The listing builds one solid part. Answer for the finished solid, in the listing's coordinates (mm). A direction names the side the tool comes from. Coordinates: 2 decimals unless noted, no trailing zeros. Loops run counter-clockwise (first coordinate to the right, second up) from the corner with the lowest first, then second, coordinate; pieces in that order, holes last. Notation, with made-up numbers: M 79.25,2 L 88.25,2 A11 ccw 88.25,8 Z; hole C 48,76 d5. An arc over 180 degrees is marked long. Return JSON: item names as keys, results as strings. Group by question number.
1. Straight lines are drawn through the part: L1, parallel to X at y = 24.9, z = 0; L2, parallel to X at y = 22.3, z = 23.57; L3, parallel to Y at x = -10.5, z = 25.5. For each, find the intervals that lie inside material, in ascending order. Write a range as from..to.
2. Given P1, Ø3, axis at x = 7.5, y = -17, coming from the +Z side; P2, Ø6, axis at x = -23.57, z = -23.57, coming from the +Y side; P3, Ø4, axis at y = 24.5, z = -6.5, coming from the +X side, each flat-ended and moving along its own axis, determine where each tip first touches the part or whether it passes through.
3. Section D-D (x = 22.5) is taken. Count the separate pieces of the cut face and the enclosed holes in it, then the cut area to 3 significant figures.
4. Section A-A (y = -8) is taken. Write down the section's boundary in (x, z), then the cut area to 3 significant figures.
5. Which of the six approach directions +Z, -Z, +X, -X, +Y, -Y give full straight-line access (tool end or side, diameter ignored) to faces 1 (the face through (20.624, 3.121, 20.532)), 2 (the face through (1.802, 25.289, 5.723)), 3 (the face through (0, -13, -31))?
6. The mould has two halves that part along X. Classify faces 4 (the face through (25.79, 22.13, 22.42)), 5 (the face through (-20.624, 3.121, -20.532)), 6 (the face through (-0.4, 24.5, -19.2)): pulls with the +X half, pulls with the -X half, needs draft (parallel to the pull), parting line crosses it, or undercut.
7. Section C-C (x = 12.5) is taken. Write down the section's boundary in (y, z), then the cut area to 3 significant figures.
```python
from build123d import *

# Parameters (mm, degrees)
SKETCH1_W                = 56.4
SKETCH1_H                = 56.4
BOSS_EXTRUDE1_DEPTH      = 24.5
CUT_EXTRUDE1_START       = 4.8
CUT_EXTRUDE1_DEPTH       = 59.378160784
FILLET1_R                = 3
FILLET2_R                = 1
SKETCH3_R                = 2.5
CUT_EXTRUDE2_DEPTH       = 55.8
SKETCH4_R                = 19.05
BOSS_EXTRUDE2_DEPTH      = 1.6
SKETCH5_R                = 3.175
BOSS_EXTRUDE3_DEPTH      = 33.5
CUT_EXTRUDE3_START       = -15
CUT_EXTRUDE3_DEPTH       = 15
CUT_EXTRUDE4_DEPTH       = 71.388067171
CUT_EXTRUDE4_DEPTH_BACK  = 71.388067171
FILLET3_R                = 5
CUT_EXTRUDE5_START       = -1.6
SKETCH8_R                = 6
SKETCH8_R_2              = 3.175
CUT_EXTRUDE5_DEPTH       = 1.6
BOSS_EXTRUDE4_START      = -11.5
BOSS_EXTRUDE4_DEPTH      = 33
BOSS_EXTRUDE5_DEPTH      = 6.4
BOSS_EXTRUDE5_DEPTH_BACK = 50.6
SKETCH11_R               = 4
BOSS_EXTRUDE6_START      = -1
SKETCH12_W               = 20.6
SKETCH12_H               = 11.5
BOSS_EXTRUDE6_DEPTH      = 6.4


with BuildPart() as part:
    # Sketch1 → Boss-Extrude1 (new, symmetric)
    with BuildSketch(Plane(origin=(0, 0, 0), x_dir=(1, 0, 0), z_dir=(0, 1, 0))):
        Rectangle(SKETCH1_W, SKETCH1_H)
    extrude(amount=BOSS_EXTRUDE1_DEPTH, both=True)

    # Sketch2 → Cut-Extrude1 (cut, through all)
    with BuildSketch(Plane.XZ.offset(-24.5).offset(CUT_EXTRUDE1_START)):
        with BuildLine():
            Line((-18.75, 28.2), (-18.75, 24.75))
            ThreePointArc((-18.75, 24.75), (-20.507359313, 20.507359313), (-24.75, 18.75))
            Line((-24.75, 18.75), (-28.2, 18.75))
            Line((-28.2, 18.75), (-28.2, 28.2))
            Line((-28.2, 28.2), (-18.75, 28.2))
        make_face()
        with BuildLine():
            Line((28.2, 28.2), (28.2, 18.75))
            Line((28.2, 18.75), (24.75, 18.75))
            ThreePointArc((24.75, 18.75), (20.507359313, 20.507359313), (18.75, 24.75))
            Line((18.75, 24.75), (18.75, 28.2))
            Line((18.75, 28.2), (28.2, 28.2))
        make_face()
        with BuildLine():
            Line((18.75, -28.2), (18.75, -24.75))
            ThreePointArc((18.75, -24.75), (20.507359313, -20.507359313), (24.75, -18.75))
            Line((24.75, -18.75), (28.2, -18.75))
            Line((28.2, -18.75), (28.2, -28.2))
            Line((28.2, -28.2), (18.75, -28.2))
        make_face()
        with BuildLine():
            Line((-28.2, -28.2), (-28.2, -18.75))
            Line((-28.2, -18.75), (-24.75, -18.75))
            ThreePointArc((-24.75, -18.75), (-20.507359313, -20.507359313), (-18.75, -24.75))
            Line((-18.75, -24.75), (-18.75, -28.2))
            Line((-18.75, -28.2), (-28.2, -28.2))
        make_face()
    extrude(amount=CUT_EXTRUDE1_DEPTH, mode=Mode.SUBTRACT)

    # Fillet1
    fillet1_edges = [part.edges().sort_by_distance(p)[0] for p in [
        (-28.2, -2.4, -18.75),
        (-18.75, -2.4, -28.2),
        (18.75, -2.4, -28.2),
        (28.2, -2.4, -18.75),
        (28.2, -2.4, 18.75),
        (18.75, -2.4, 28.2),
        (-18.75, -2.4, 28.2),
        (-28.2, -2.4, 18.75),
        (28.2, 22.1, 28.2),
        (-28.2, 22.1, 28.2),
        (-28.2, 22.1, -28.2),
        (28.2, 22.1, -28.2),
    ]]
    fillet(fillet1_edges, radius=FILLET1_R)

    # Fillet2
    fillet2_edges = [part.edges().sort_by_distance(p)[0] for p in [
        (-20.507359313, -24.5, -20.507359313),
        (-24.975, -24.5, -18.75),
        (20.507359313, -24.5, -20.507359313),
        (18.75, -24.5, -24.975),
        (20.507359313, -24.5, 20.507359313),
        (24.975, -24.5, 18.75),
        (-20.507359313, -24.5, 20.507359313),
        (-18.75, -24.5, 24.975),
        (-28.2, -24.5, 0),
        (-18.75, -24.5, -24.975),
        (0, -24.5, -28.2),
        (24.975, -24.5, -18.75),
        (28.2, -24.5, 0),
        (18.75, -24.5, 24.975),
        (0, -24.5, 28.2),
        (-24.975, -24.5, 18.75),
        (-17.871320344, -24.5, 27.321320344),
        (-17.871320344, -24.5, -27.321320344),
        (17.871320344, -24.5, -27.321320344),
        (27.321320344, -24.5, -17.871320344),
        (27.321320344, -24.5, 17.871320344),
        (17.871320344, -24.5, 27.321320344),
        (-27.321320344, -24.5, 17.871320344),
        (-27.321320344, -24.5, -17.871320344),
    ]]
    fillet(fillet2_edges, radius=FILLET2_R)

    # Sketch3 → Cut-Extrude2 (cut)
    with BuildSketch(Plane(origin=(0, 24.5, 0), x_dir=(1, 0, 0), z_dir=(0, 1, 0))):
        with Locations(Location((23.57, 23.57, 0), (0, 0, 270))):
            Circle(SKETCH3_R)
        with Locations(Location((-23.57, 23.57, 0), (0, 0, 90))):
            Circle(SKETCH3_R)
        with Locations(Location((23.57, -23.57, 0), (0, 0, 90))):
            Circle(SKETCH3_R)
        with Locations(Location((-23.57, -23.57, 0), (0, 0, 270))):
            Circle(SKETCH3_R)
    extrude(amount=-CUT_EXTRUDE2_DEPTH, mode=Mode.SUBTRACT)

    # Sketch4 → Boss-Extrude2 (add)
    with BuildSketch(Plane(origin=(0, 24.5, 0), x_dir=(1, 0, 0), z_dir=(0, 1, 0))):
        with Locations(Location((0, 0, 0), (0, 0, 270))):
            Circle(SKETCH4_R)
    extrude(amount=BOSS_EXTRUDE2_DEPTH)

    # Sketch5 → Boss-Extrude3 (add)
    with BuildSketch(Plane(origin=(0, 24.5, 0), x_dir=(1, 0, 0), z_dir=(0, 1, 0))):
        with Locations(Location((0, 0, 0), (0, 0, 270))):
            Circle(SKETCH5_R)
    extrude(amount=BOSS_EXTRUDE3_DEPTH)

    # Sketch6 → Cut-Extrude3 (cut)
    with BuildSketch(Plane(origin=(0, 58, 0), x_dir=(1, 0, 0), z_dir=(0, 1, 0)).offset(CUT_EXTRUDE3_START)):
        with BuildLine():
            Line((-2.049390153, 2.425), (2.049390153, 2.425))
            ThreePointArc((2.049390153, 2.425), (0, 3.175), (-2.049390153, 2.425))
        make_face()
    extrude(amount=CUT_EXTRUDE3_DEPTH, mode=Mode.SUBTRACT)

    # Sketch7 → Cut-Extrude4 (cut, two sides: drawn at the far end of the back side and taken through both)
    with BuildSketch(Plane(origin=(0, 0, 0), x_dir=(0, 0, -1), z_dir=(1, 0, 0)).offset(-CUT_EXTRUDE4_DEPTH_BACK)):
        Polygon((2.425, 43), (3.175, 41), (3.175, 43), align=None)
    extrude(amount=CUT_EXTRUDE4_DEPTH + CUT_EXTRUDE4_DEPTH_BACK, mode=Mode.SUBTRACT)

    # Fillet3
    fillet3_edges = [part.edges().sort_by_distance(p)[0] for p in [
        (0, 43, -2.425),
    ]]
    fillet(fillet3_edges, radius=FILLET3_R)

    # Sketch8 → Cut-Extrude5 (cut)
    with BuildSketch(Plane(origin=(0, 26.1, 0), x_dir=(1, 0, 0), z_dir=(0, 1, 0)).offset(CUT_EXTRUDE5_START)):
        with Locations(Location((0, 0, 0), (0, 0, 270))):
            Circle(SKETCH8_R)
        with Locations(Location((0, 0, 0), (0, 0, 59.774237817))):
            Circle(SKETCH8_R_2, mode=Mode.SUBTRACT)
    extrude(amount=CUT_EXTRUDE5_DEPTH, mode=Mode.SUBTRACT)

    # Sketch11 → Boss-Extrude5 (add, two sides: drawn at the far end of the back side and taken through both)
    with BuildSketch(Plane(origin=(0, 26.1, 0), x_dir=(1, 0, 0), z_dir=(0, 1, 0)).offset(-BOSS_EXTRUDE5_DEPTH_BACK)):
        with Locations(Location((0, 0, 0), (0, 0, 270))):
            Circle(SKETCH11_R)
    extrude(amount=BOSS_EXTRUDE5_DEPTH + BOSS_EXTRUDE5_DEPTH_BACK)



with BuildPart() as body_2:
    # Sketch10 → Boss-Extrude4 (new body)
    with BuildSketch(Plane.XZ.offset(24.5).offset(BOSS_EXTRUDE4_START)):
        with BuildLine():
            Line((25.2, 18.85), (24.75, 18.85))
            ThreePointArc((24.75, 18.85), (20.578069991, 20.578069991), (18.85, 24.75))
            Line((18.85, 24.75), (18.85, 25.2))
            ThreePointArc((18.85, 25.2), (17.942031022, 27.392031022), (15.75, 28.3))
            Line((15.75, 28.3), (-15.75, 28.3))
            ThreePointArc((-15.75, 28.3), (-17.942031022, 27.392031022), (-18.85, 25.2))
            Line((-18.85, 25.2), (-18.85, 24.75))
            ThreePointArc((-18.85, 24.75), (-20.578069991, 20.578069991), (-24.75, 18.85))
            Line((-24.75, 18.85), (-25.2, 18.85))
            ThreePointArc((-25.2, 18.85), (-27.392031022, 17.942031022), (-28.3, 15.75))
            Line((-28.3, 15.75), (-28.3, -15.75))
            ThreePointArc((-28.3, -15.75), (-27.392031022, -17.942031022), (-25.2, -18.85))
            Line((-25.2, -18.85), (-24.75, -18.85))
            ThreePointArc((-24.75, -18.85), (-20.578069991, -20.578069991), (-18.85, -24.75))
            Line((-18.85, -24.75), (-18.85, -25.2))
            ThreePointArc((-18.85, -25.2), (-17.942031022, -27.392031022), (-15.75, -28.3))
            Line((-15.75, -28.3), (15.75, -28.3))
            ThreePointArc((15.75, -28.3), (17.942031022, -27.392031022), (18.85, -25.2))
            Line((18.85, -25.2), (18.85, -24.75))
            ThreePointArc((18.85, -24.75), (20.578069991, -20.578069991), (24.75, -18.85))
            Line((24.75, -18.85), (25.2, -18.85))
            ThreePointArc((25.2, -18.85), (27.392031022, -17.942031022), (28.3, -15.75))
            Line((28.3, -15.75), (28.3, 15.75))
            ThreePointArc((28.3, 15.75), (27.392031022, 17.942031022), (25.2, 18.85))
        make_face()
        with BuildLine():
            Line((28.2, -15.75), (28.2, 15.75))
            ThreePointArc((28.2, 15.75), (27.321320344, 17.871320344), (25.2, 18.75))
            Line((25.2, 18.75), (24.75, 18.75))
            ThreePointArc((24.75, 18.75), (20.507359313, 20.507359313), (18.75, 24.75))
            Line((18.75, 24.75), (18.75, 25.2))
            ThreePointArc((18.75, 25.2), (17.871320344, 27.321320344), (15.75, 28.2))
            Line((15.75, 28.2), (-15.75, 28.2))
            ThreePointArc((-15.75, 28.2), (-17.871320344, 27.321320344), (-18.75, 25.2))
            Line((-18.75, 25.2), (-18.75, 24.75))
            ThreePointArc((-18.75, 24.75), (-20.507359313, 20.507359313), (-24.75, 18.75))
            Line((-24.75, 18.75), (-25.2, 18.75))
            ThreePointArc((-25.2, 18.75), (-27.321320344, 17.871320344), (-28.2, 15.75))
            Line((-28.2, 15.75), (-28.2, -15.75))
            ThreePointArc((-28.2, -15.75), (-27.321320344, -17.871320344), (-25.2, -18.75))
            Line((-25.2, -18.75), (-24.75, -18.75))
            ThreePointArc((-24.75, -18.75), (-20.507359313, -20.507359313), (-18.75, -24.75))
            Line((-18.75, -24.75), (-18.75, -25.2))
            ThreePointArc((-18.75, -25.2), (-17.871320344, -27.321320344), (-15.75, -28.2))
            Line((-15.75, -28.2), (15.75, -28.2))
            ThreePointArc((15.75, -28.2), (17.871320344, -27.321320344), (18.75, -25.2))
            Line((18.75, -25.2), (18.75, -24.75))
            ThreePointArc((18.75, -24.75), (20.507359313, -20.507359313), (24.75, -18.75))
            Line((24.75, -18.75), (25.2, -18.75))
            ThreePointArc((25.2, -18.75), (27.321320344, -17.871320344), (28.2, -15.75))
        make_face(mode=Mode.SUBTRACT)
    extrude(amount=-BOSS_EXTRUDE4_DEPTH)


with BuildPart() as part_1:
    add(part.part)

    add(body_2.part)  # Boss-Extrude6 merges body 2
    # Sketch12 → Boss-Extrude6 (add)
    with BuildSketch(Plane(origin=(0, 0, -28.2), x_dir=(-1, 0, 0), z_dir=(0, 0, -1)).offset(BOSS_EXTRUDE6_START)):
        with Locations((0, -18.75)):
            Rectangle(SKETCH12_W, SKETCH12_H)
    extrude(amount=BOSS_EXTRUDE6_DEPTH)


solid = part_1.part
```
Worked out:
{
 "1": {"L1": "-19.05..-6, -4..4, 6..19.05", "L2": "-28.2..-26.07, -21.07..21.07, 26.07..28.2", "L3": "-24.5..24.5"},
 "2": {"P1": "z = 28.2", "P2": "y = 24.5", "P3": "x = 28.2"},
 "3": {"separate pieces": "3", "enclosed holes": "0", "area": "1,930 mm^2"},
 "4": {"outline": "M -28.3,-15.75 A3.1 ccw -25.2,-18.85 L -24.75,-18.85 A5.9 cw -18.85,-24.75 L -18.85,-25.2 A3.1 ccw -15.75,-28.3 L 15.75,-28.3 A3.1 ccw 18.85,-25.2 L 18.85,-24.75 A5.9 cw 24.75,-18.85 L 25.2,-18.85 A3.1 ccw 28.3,-15.75 L 28.3,15.75 A3.1 ccw 25.2,18.85 L 24.75,18.85 A5.9 cw 18.85,24.75 L 18.85,25.2 A3.1 ccw 15.75,28.3 L -15.75,28.3 A3.1 ccw -18.85,25.2 L -18.85,24.75 A5.9 cw -24.75,18.85 L -25.2,18.85 A3.1 ccw -28.3,15.75 Z", "area": "2,860 mm^2"},
 "5": {"face 1": "+Z, +X, -Y", "face 2": "+Y", "face 3": "-Z, +X, -X, +Y"},
 "6": {"face 4": "undercut", "face 5": "pulls with the -X half", "face 6": "needs draft"},
 "7": {"outline": "M -24.5,-27.2 A1 ccw -23.5,-28.2 L -13,-28.2 L -13,-28.3 L 20,-28.3 L 20,-28.2 L 24.5,-28.2 L 24.5,-14.38 L 26.1,-14.38 L 26.1,14.38 L 24.5,14.38 L 24.5,28.2 L 20,28.2 L 20,28.3 L -13,28.3 L -13,28.2 L -23.5,28.2 A1 ccw -24.5,27.2 Z", "area": "2,820 mm^2"}
}
